The figure shows three views and two pictorial views of one solid part (mm, origin at its lowest corner). Answer the questions. A direction names the side the tool comes from. Coordinates: 2 decimals unless noted, no trailing zeros. Order: outer loops, then holes, each group sorted by start corner. A loop starts at its lowest first (then second) coordinate and runs counter-clockwise, first axis right, second up. Notation, with made-up numbers: (-8.75, -3) -> (9.25, -3) arc R25 cw to (9.25, 36) -> close; hole circle Ø2 at (40.25, 8.5). An arc over 180 degrees is marked (long way). Return JSON: item names as keys, results as strings.
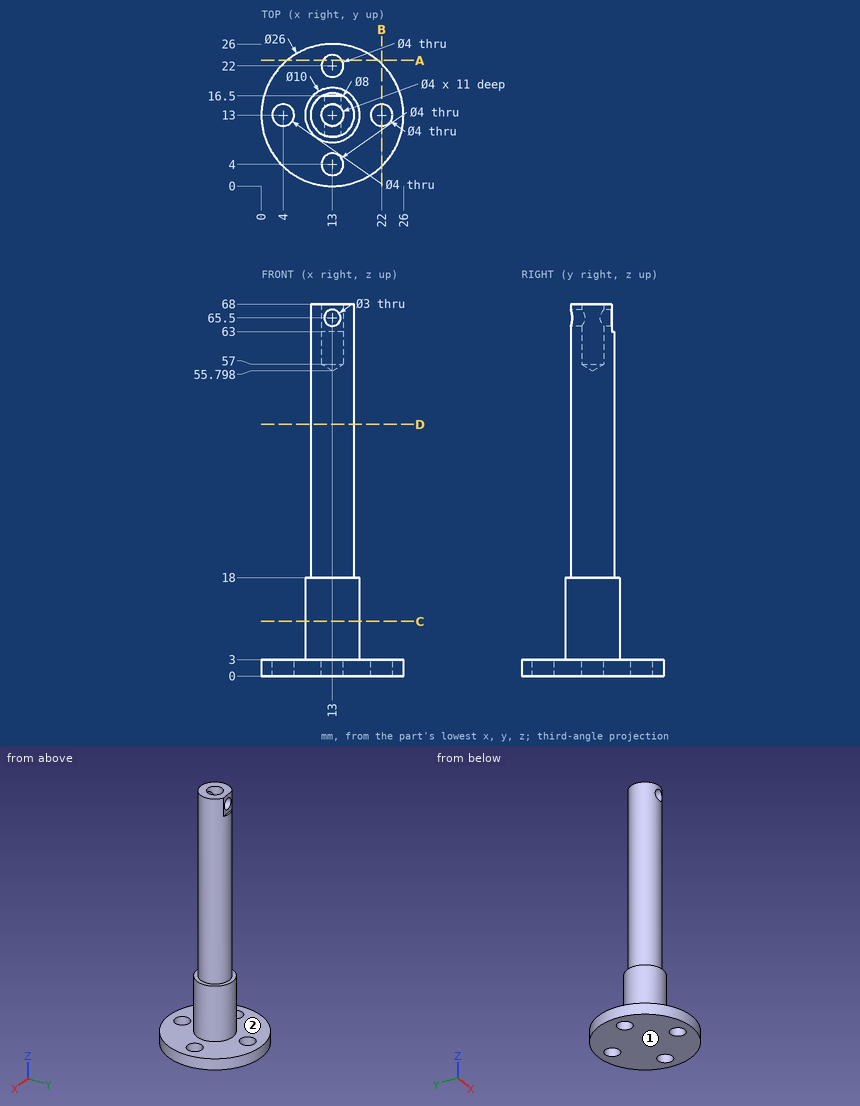
Item 1: Find the intervals of material crossed by probe 1 along Z at (x, y) = (3.5, 6.5); probe 2 along Z at (x, y) = (11, 8.5); probe 3 along X at (y, z) = (10.1, 65.5) (1 decimal), in increasing order.
Answer list:
{"probe 1": "0 to 3", "probe 2": "0 to 18", "probe 3": "10.2 to 11.5, 14.5 to 15.8"}
Item 2: Flat-ended cylindrical pins translate along their axes: pin 1 (2.5 mm diameter, centred on x = 13, y = 22, fed in from +Z); pin 2 (4.5 mm diameter, centred on x = 13, z = 66, fed in from +Y); pin 3 (10 mm diameter, centred on y = 20, z = 28.5, fed in from +X); pin 4 (2 mm diameter, centred on y = 13.5, z = 27, fed in from -X). Find the tip coordinate at first contact, or state that the pin passes through.
Answer list:
{"pin 1": "through", "pin 2": "y = 16.5", "pin 3": "x = 16.46", "pin 4": "x = 9"}
Item 3: The part is cut by section A-A on y = 23. Determine the outline of the cut face in (x, z).
Answer list:
{"outline": "(4.69, 0) -> (11.27, 0) -> (11.27, 3) -> (4.69, 3) -> close; (14.73, 0) -> (21.31, 0) -> (21.31, 3) -> (14.73, 3) -> close"}
Item 4: Which of the six approach directions +Z, -Z, +X, -X, +Y, -Y give full straight-line access (tool end or side, diameter ignored) to the marked faces 1 and 2?
Answer list:
{"face 1": "-Z, +X, -X, +Y, -Y", "face 2": "+Z"}
Item 5: The part is cut by section B-B on x = 22. Determine the outline of the cut face in (y, z), plus the area to 3 significant figures.
Answer list:
{"outline": "(3.62, 0) -> (11, 0) -> (11, 3) -> (3.62, 3) -> close; (15, 0) -> (22.38, 0) -> (22.38, 3) -> (15, 3) -> close", "area": "44.3 mm2"}
Item 6: The part is cut by section D-D on z = 46. Determine the outline of the cut face in (x, y), plus the area to 3 significant figures.
Answer list:
{"outline": "circle Ø8 at (13, 13)", "area": "50.3 mm2"}
Item 7: The part is cut by section C-C on z = 10. Determine the outline of the cut face in (x, y).
Answer list:
{"outline": "circle Ø10 at (13, 13)"}
